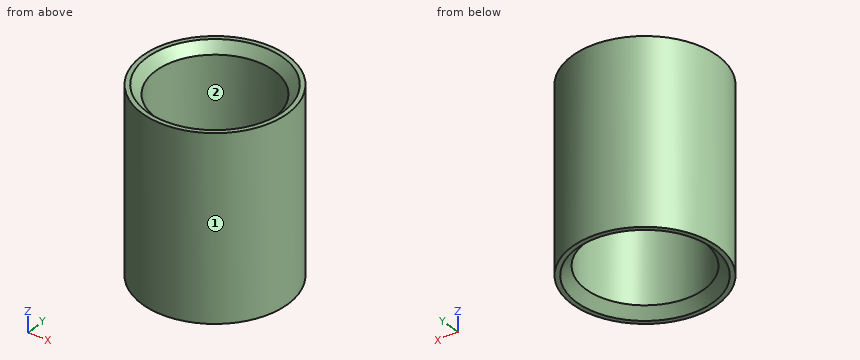
from build123d import *

# Parameters (mm, degrees)
SKETCH_R        = 8
SKETCH_R_2      = 6.5
PAD_DEPTH       = 20
CHAMFER_SIZE    = 1
CHAMFER001_SIZE = 1


with BuildPart() as part:
    # Sketch → Pad (new body)
    with BuildSketch(Plane.XY):
        Circle(SKETCH_R)
        Circle(SKETCH_R_2, mode=Mode.SUBTRACT)
    extrude(amount=PAD_DEPTH)

    # Chamfer
    chamfer_edges = [part.edges().sort_by_distance(p)[0] for p in [
        (-6.5, 0, 20),
    ]]
    chamfer(chamfer_edges, length=CHAMFER_SIZE)

    # Chamfer001
    chamfer001_edges = [part.edges().sort_by_distance(p)[0] for p in [
        (-6.5, 0, 0),
    ]]
    chamfer(chamfer001_edges, length=CHAMFER001_SIZE)


solid = part.part
The listing builds one solid part. Answer for the finished solid, in the listing's coordinates (mm). Face numbers are marked on the shaded views. Coordinates: 2 decimals unless noted, no trailing zeros. Write each loop counter-clockwise with the first axis right and the second up, starting at its lowest first coordinate (ties: lowest second). Pieces come first, ordered by that corner, then holes. Notation, with made-up numbers: M -30,66.25 L 1,66.25 A21 ccw 1,80.25 Z; hole C 51,73.25 d7. An arc over 180 degrees is marked long. Put each result on its own line as item: value. Start each with the question number.
1. A cutting plane is placed at A-A on y = 0. Write down the section's boundary in (x, z).
2. A cutting plane is placed at C-C on z = 14.5. Write down the section's boundary in (x, y), then the cut area to 3 significant figures.
3. Flat-ended cylindrical pins translate along their axes: P1, Ø6, axis at x = -1, z = 17.5, coming from the +Y side; P2, Ø5, axis at x = -3, y = -2.5, coming from the -Z side; P3, Ø8, axis at y = 6, z = 8.5, coming from the -X side; P4, Ø3, axis at x = -2.5, z = 2.5, coming from the -Y side. Find the tip coordinate at first contact, or state that the pin passes through.
4. For a pull along Y with two mould halves and no side action, classify the marked faces 1 and 2 as pulls with the +Y half, pulls with the -Y half, needs draft (parallel to the pull), parting line crosses it, or undercut.
5. Consider line 1 (Y direction, x = 0, z = 4.5); line 2 (X direction, y = 1.5, z = 3.75); line 3 (Y direction, x = 3.5, z = 13.75). Determine where each line is inside the solid, lowest interval first. Write a range as from..to.
Resolved:
1. outline: M -8,0 L -7.5,0 L -6.5,1 L -6.5,19 L -7.5,20 L -8,20 Z; M 6.5,1 L 7.5,0 L 8,0 L 8,20 L 7.5,20 L 6.5,19 Z
2. outline: C 0,0 d16; hole C 0,0 d13
2. area: 68.3 mm2
3. P1: stops at y = 8
3. P2: passes through
3. P3: stops at x = -7.75
3. P4: stops at y = -7.94
4. face 1: parting line crosses it
4. face 2: undercut
5. line 1: y = -8..-6.5, 6.5..8
5. line 2: x = -7.86..-6.32, 6.32..7.86
5. line 3: y = -7.19..-5.48, 5.48..7.19
